Part model, mm, in its own coordinate system. A direction names the side the tool comes from. Give positions to 0.01 mm unless a question says otherwise; leave off trailing zeros. Order: outer loops, then holes, each group sorted by start corner. A loop starts at its lowest first (then second) coordinate and runs counter-clockwise, first axis right, second up. Notation, with made-up numbers: (84, 59.25) - (90, 59.25) arc R18 ccw to (90, 81.25) - close; hole circle Ø1 at (-4, 79). An arc over 180 degrees is marked (long way). One line per item, written item: value.
Autodesk Inventor part; units mm, degrees
ref_plane "YZ Plane" through (0, 0, 0) normal (1, 0, 0) x (0, 1, 0)
ref_plane "XZ Plane" through (0, 0, 0) normal (0, 1, 0) x (-1, 0, 0)
ref_plane "XY Plane" through (0, 0, 0) normal (0, 0, 1) x (1, 0, 0)
sketch "Sketch1" plane through (0, 0, 0) normal (0, 1, 0) x (-1, 0, 0)
  circle A0 centre (0, 0) radius 3.175
  dimension "d0" = 6.35
extrude "Extrusion1" add sketch "Sketch1" along normal blind 50.8
sketch "Sketch2" plane through (0, 50.8, 0) normal (0, 1, 0) x (1, 0, 0)
  circle A0 centre (0, 0) radius 3.175
  line L0 (-5.5563, -3.2079) -> (-5.5563, 3.2079)
  line L1 (-5.5563, 3.2079) -> (0, 6.4158)
  line L2 (0, 6.4158) -> (5.5563, 3.2079)
  line L3 (5.5563, 3.2079) -> (5.5563, -3.2079)
  line L4 (5.5563, -3.2079) -> (0, -6.4158)
  line L5 (0, -6.4158) -> (-5.5563, -3.2079)
  dimension "d3" = 11.1125
  dimension "d4" = 11.1125
  dimension "d5" = 11.1125
  dimension "d6" = 120
  dimension "d7" = 120
  dimension "d8" = 5.5563
  dimension "d9" = 5.5563
  dimension "d10" = 5.5563
extrude "Extrusion2" add sketch "Sketch2" along normal blind 3.9688 contours A0 | L0 L1 L2 L3 L4 L5
thread "Thread1"
properties part number "beam breaker bolt" material "Steel, Alloy"
1) Slice it at D-D on x = 3.75. Write the cut outline in (y, z), then the cut area to 3 significant figures.
Answer:
outline: (50.8, -4.25) - (54.77, -4.25) - (54.77, 4.25) - (50.8, 4.25) - close
area: 33.7 mm2
2) Which spindle directions (+Z, -Z, +X, -X, +Y, -Y) get a long thin tool onto all of the face, cutting with end or side? Do faces 1 (the face through (-3, 50.8, 3)), 2 (the face through (-5.556, 53, 0)). Say none if no direction does.
Answer:
face 1: -Y
face 2: +Z, -Z, -X, +Y, -Y
3) Drop flat-ended pins along their axis: P1, Ø3, axis at y = 46, z = -1, coming from the +X side (3 decimals); P2, Ø2, axis at y = 41.5, z = 4.5, coming from the +X side; P3, Ø3, axis at x = -4, y = 10, coming from the -Z side; P4, Ø4, axis at x = -1, y = 26.5, coming from the +Z side (3 decimals). Give the stop position or say it passes through.
Answer:
P1: stops at x = 3.175
P2: passes through
P3: stops at z = -1.96
P4: stops at z = 3.175
4) Wall check: line 1 along Y through (x, z) = (0.5, -4.5); line 2 along Z through (x, y) = (-0.25, 33); line 3 along Z through (x, y) = (0.75, 52.5). Give the ranges that are in metal, low to high. Write a range as [from, to].
Answer:
line 1: y = [50.8, 54.77]
line 2: z = [-3.17, 3.17]
line 3: z = [-5.98, 5.98]
5) Slice it at C-C on y = 50. Write the cut outline in (x, z) (3 decimals).
Answer:
outline: circle Ø6.35 at (0, 0)
6) Slice it at B-B on x = 0.5. Write the cut outline in (y, z).
Answer:
outline: (0, -3.14) - (50.8, -3.14) - (50.8, -6.13) - (54.77, -6.13) - (54.77, 6.13) - (50.8, 6.13) - (50.8, 3.14) - (0, 3.14) - close
7) Slice it at A-A on z = 0. Write the cut outline in (x, y) (3 decimals).
Answer:
outline: (-5.556, 50.8) - (-3.175, 50.8) - (-3.175, 0) - (3.175, 0) - (3.175, 50.8) - (5.556, 50.8) - (5.556, 54.769) - (-5.556, 54.769) - close
